from build123d import *

# Parameters (mm, degrees)
SKETCH1_W           = 30
SKETCH1_H           = 16
BOSS_EXTRUDE1_DEPTH = 8.5
SKETCH2_R           = 4.5
CUT_EXTRUDE1_DEPTH  = 5.2
SKETCH3_R           = 2.65
CUT_EXTRUDE2_DEPTH  = 35.395348523
CUT_EXTRUDE3_DEPTH  = 14
SKETCH5_R           = 2.1
CUT_EXTRUDE4_DEPTH  = 7
SKETCH6_R           = 1.1
CUT_EXTRUDE5_DEPTH  = 2.5


with BuildPart() as part:
    # Sketch1 → Boss-Extrude1 (new body)
    with BuildSketch(Plane(origin=(0, 0, 0), x_dir=(1, 0, 0), z_dir=(0, 1, 0))):
        with Locations((15, 8)):
            Rectangle(SKETCH1_W, SKETCH1_H)
    extrude(amount=BOSS_EXTRUDE1_DEPTH)

    # Sketch2 → Cut-Extrude1 (cut)
    with BuildSketch(Plane(origin=(0, 8.5, 0), x_dir=(1, 0, 0), z_dir=(0, 1, 0))):
        with Locations(Location((15, 7, 0), (0, 0, 270))):
            Circle(SKETCH2_R)
    extrude(amount=-CUT_EXTRUDE1_DEPTH, mode=Mode.SUBTRACT)

    # Sketch3 → Cut-Extrude2 (cut, through all)
    with BuildSketch(Plane(origin=(0, 3.3, 0), x_dir=(1, 0, 0), z_dir=(0, 1, 0))):
        with Locations(Location((15, 7, 0), (0, 0, 270))):
            Circle(SKETCH3_R)
    extrude(amount=-CUT_EXTRUDE2_DEPTH, mode=Mode.SUBTRACT)

    # Sketch4 → Cut-Extrude3 (cut)
    with BuildSketch(Plane(origin=(0, 0, -16), x_dir=(-1, 0, 0), z_dir=(0, 0, -1))):
        Polygon((-27, 8.5), (-24.68995278, 4.498880847), (-30, 4.498880847), (-30, 8.5), align=None)
        Polygon((0, 8.5), (-3, 8.5), (-5.31004722, 4.498880847), (0, 4.498880847), align=None)
    extrude(amount=-CUT_EXTRUDE3_DEPTH, mode=Mode.SUBTRACT)

    # Sketch5 → Cut-Extrude4 (cut)
    with BuildSketch(Plane(origin=(0, 0, -16), x_dir=(-1, 0, 0), z_dir=(0, 0, -1))):
        with Locations((-21.5, 4.25)):
            Circle(SKETCH5_R)
        with Locations(Location((-8.5, 4.25, 0), (0, 0, 180))):
            Circle(SKETCH5_R)
    extrude(amount=-CUT_EXTRUDE4_DEPTH, mode=Mode.SUBTRACT)

    # Sketch6 → Cut-Extrude5 (cut)
    with BuildSketch(Plane.XZ):
        with Locations(Location((10.119225975, -7, 0), (0, 0, 270))):
            Circle(SKETCH6_R)
        with Locations(Location((19.880774025, -7, 0), (0, 0, 270))):
            Circle(SKETCH6_R)
    extrude(amount=-CUT_EXTRUDE5_DEPTH, mode=Mode.SUBTRACT)


solid = part.part
Could you check a few things on this model? Use its own coordinates, in mm. A direction names the side the tool comes from. Coordinates: 2 decimals unless noted, no trailing zeros. Loops run counter-clockwise (first coordinate to the right, second up) from the corner with the lowest first, then second, coordinate; pieces in that order, holes last. Notation, with made-up numbers: (-8.75, 2) -> (47.25, 2) arc R19 cw to (47.25, 17) -> close; hole circle Ø1 at (2, 6). An arc over 180 degrees is marked (long way). Answer in a Markdown table with one row per item.
(1) Imagine slicing it at C-C (x = 8.5). List the corners of the cut face in (y, z) for me.
Results found:
| item | result |
|---|---|
| outline | (0, -16) -> (2.15, -16) -> (2.15, -9) -> (6.35, -9) -> (6.35, -16) -> (8.5, -16) -> (8.5, 0) -> (0, 0) -> close |
(2) If I drill on probe 1 along X at (y, z) = (1.95, -7); probe 2 along Z at (x, y) = (19.75, 1); probe 3 along Y at (x, z) = (8.5, -12.75), over which ranges is the centre line in solid material (lowest first)?
Results found:
| item | result |
|---|---|
| probe 1 | x = 0 to 9.02, 11.22 to 12.35, 17.65 to 18.78, 20.98 to 30 |
| probe 2 | z = -16 to -8.09, -5.91 to 0 |
| probe 3 | y = 0 to 2.15, 6.35 to 8.5 |
(3) Imagine slicing it at D-D (z = -13.5). List the corners of the cut face in (x, y) for me, plus the area to 3 significant figures.
Results found:
| item | result |
|---|---|
| outline | (0, 0) -> (30, 0) -> (30, 4.5) -> (24.69, 4.5) -> (27, 8.5) -> (3, 8.5) -> (5.31, 4.5) -> (0, 4.5) -> close; hole circle Ø4.2 at (8.5, 4.25); hole circle Ø4.2 at (21.5, 4.25) |
| area | 194 mm^2 |
(4) For faces 5 (the face through (15, 0, -10)), 6 (the face through (28, 7, -2)), 7 (the face through (20.97, 1.23, -6.86)), 8 (the face through (8, 4, -9)), 9 (the face through (4.139, 6.527, -9.098)), which set-ups out of +Z, -Z, +X, -X, +Y, -Y let a thin tool reach every point of the face, with its end or its side?
Results found:
| item | result |
|---|---|
| face 5 | +Z, -Z, +X, -X, -Y |
| face 6 | -Z, +X |
| face 7 | -Y |
| face 8 | -Z |
| face 9 | -Z, -X |
(5) Will these pins go through, and if not, where does the flat tip stop? pin 1 Ø2 at (x, y) = (21.5, 5) entering from -Z; pin 2 Ø1.1 at (x, z) = (19.5, -7) entering from -Y; pin 3 Ø4.5 at (x, z) = (15.5, -7) entering from +Y.
Results found:
| item | result |
|---|---|
| pin 1 | stops at z = -9 |
| pin 2 | stops at y = 2.5 |
| pin 3 | stops at y = 3.3 |
(6) Imagine slicing it at A-A (z = -7). List the corners of the cut face in (x, y) for me, plus the area to 3 significant figures.
Results found:
| item | result |
|---|---|
| outline | (0, 0) -> (9.02, 0) -> (9.02, 2.5) -> (11.22, 2.5) -> (11.22, 0) -> (12.35, 0) -> (12.35, 3.3) -> (10.5, 3.3) -> (10.5, 8.5) -> (3, 8.5) -> (5.31, 4.5) -> (0, 4.5) -> close; (17.65, 0) -> (18.78, 0) -> (18.78, 2.5) -> (20.98, 2.5) -> (20.98, 0) -> (30, 0) -> (30, 4.5) -> (24.69, 4.5) -> (27, 8.5) -> (19.5, 8.5) -> (19.5, 3.3) -> (17.65, 3.3) -> close |
| area | 146 mm^2 |
(7) Thinking about a two-plate mould opening in Y: for faces 1 (the face through (18.794, 5.936, -4.581)), 2 (the face through (22, 4, -9)), 3 (the face through (13, 3.3, -5)), 4 (the face through (10, 2.5, -7)), which applies, released by +Y, released by -Y, zero draft, split by the parting line, or undercut?
Results found:
| item | result |
|---|---|
| face 1 | zero draft |
| face 2 | undercut |
| face 3 | released by +Y |
| face 4 | released by -Y |
(8) Imagine slicing it at B-B (x = 15). List the corners of the cut face in (y, z) for me.
Results found:
| item | result |
|---|---|
| outline | (0, -16) -> (8.5, -16) -> (8.5, -11.5) -> (3.3, -11.5) -> (3.3, -9.65) -> (0, -9.65) -> close; (0, -4.35) -> (3.3, -4.35) -> (3.3, -2.5) -> (8.5, -2.5) -> (8.5, 0) -> (0, 0) -> close |
